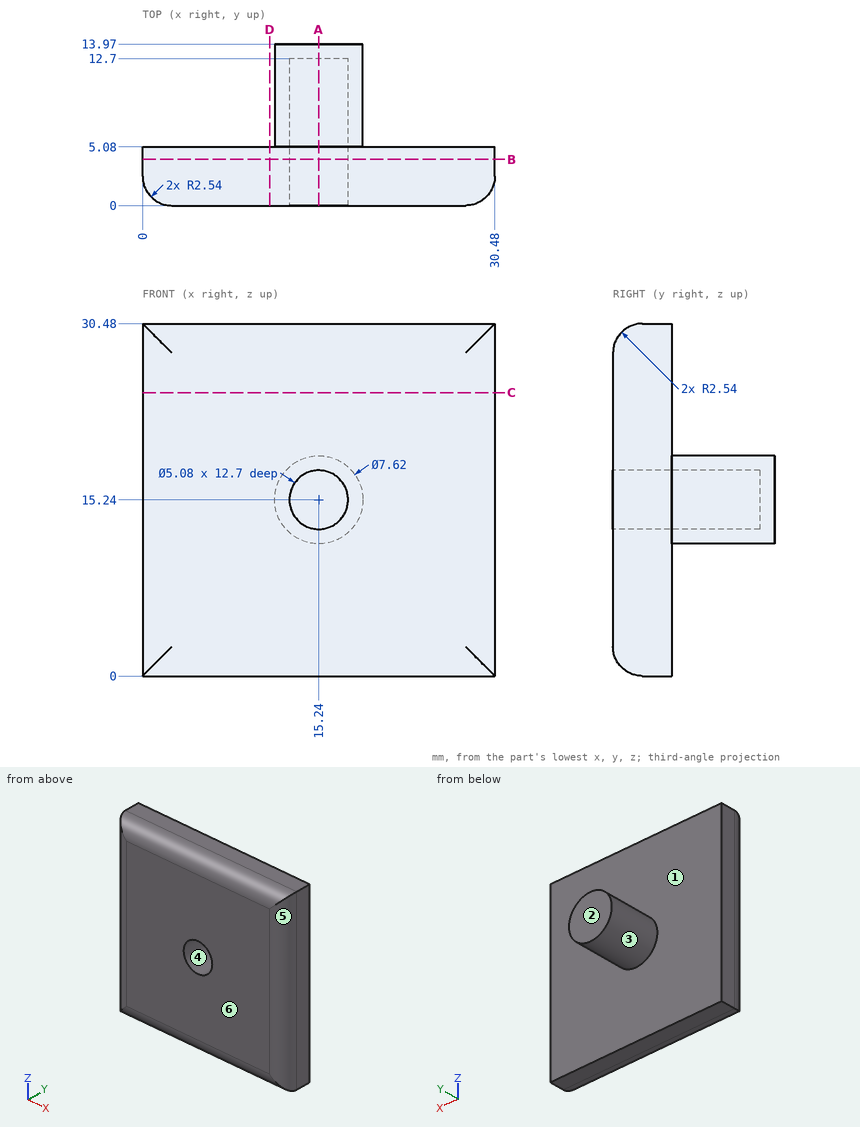
For this review, use the dimensioned drawing (mm, ordinates from the lowest corner) and the shaded views. A direction names the side the tool comes from. Round coordinates to 2 decimals unless told otherwise and drop trailing zeros. Order: outer loops, then holes, each group sorted by start corner. A loop starts at its lowest first (then second) coordinate and runs counter-clockwise, first axis right, second up. Notation, with made-up numbers: M 51.25,1 L 62.25,1 A9 ccw 62.25,13 Z; hole C -40,-24.5 d8. An arc over 180 degrees is marked long. Use a Markdown table: item, result. Add a question column.
Item 1: Insertion check: pin 1 (8 mm diameter, centred on y = 7.5, z = 21.5, fed in from +X); pin 2 (2 mm diameter, centred on y = 11, z = 17.5, fed in from +X); pin 3 (5 mm diameter, centred on x = 3, z = 4, fed in from +Y). Each pin has a flat end and moves straight along its axis. Give the tip position at first contact, or say it passes through.
Item 2: Add section B-B, the plane y = 4. Give the boundary of the cut face in (x, z), then the cut area to 3 significant figures.
Item 3: Add section D-D, the plane x = 11. Give the boundary of the cut face in (y, z).
Item 4: Tool access review of the marked faces 1 and 2: name each direction out of +Z, -Z, +X, -X, +Y, -Y from which nothing blocks a thin tool from reaching the whole face with its end or side.
Item 5: Mouldability with a two-part tool opening along X and no side actions: class the marked faces 3, 4, 5 and 6 as released by +X, released by -X, zero draft, split by the parting line, or undercut.
Item 6: Add section C-C, the plane z = 24.5. Give the boundary of the cut face in (x, y).
Item 7: To check wall thickness, follow line 1 along Z through (x, y) = (15.24, 8.5); line 2 along Y through (x, z) = (6.5, 20.5); line 3 along Z through (x, y) = (13.5, 12.5). State the ranges of each line that lie inside material, in increasing order.
Item 8: Add section A-A, the plane x = 15.24. Give the boundary of the cut face in (y, z), then the cut area to 3 significant figures.
Geometry results:
| question | item | result |
|---|---|---|
| 1 | pin 1 | stops at x = 30.48 |
| 1 | pin 2 | stops at x = 18.84 |
| 1 | pin 3 | stops at y = 5.08 |
| 2 | outline | M 0,0 L 30.48,0 L 30.48,30.48 L 0,30.48 Z; hole C 15.24,15.24 d5.08 |
| 2 | area | 909 mm² |
| 3 | outline | M 0,2.54 A2.54 ccw 2.54,0 L 5.08,0 L 5.08,30.48 L 2.54,30.48 A2.54 ccw 0,27.94 Z |
| 4 | face 1 | +Y |
| 4 | face 2 | +Z, -Z, +X, -X, +Y |
| 5 | face 3 | split by the parting line |
| 5 | face 4 | undercut |
| 5 | face 5 | released by +X |
| 5 | face 6 | zero draft |
| 6 | outline | M 0,2.54 A2.54 ccw 2.54,0 L 27.94,0 A2.54 ccw 30.48,2.54 L 30.48,5.08 L 0,5.08 Z |
| 7 | line 1 | z = 11.43 to 12.7, 17.78 to 19.05 |
| 7 | line 2 | y = 0 to 5.08 |
| 7 | line 3 | z = 11.85 to 13.39, 17.09 to 18.63 |
| 8 | outline | M 0,2.54 A2.54 ccw 2.54,0 L 5.08,0 L 5.08,11.43 L 13.97,11.43 L 13.97,19.05 L 5.08,19.05 L 5.08,30.48 L 2.54,30.48 A2.54 ccw 0,27.94 L 0,17.78 L 12.7,17.78 L 12.7,12.7 L 0,12.7 Z |
| 8 | area | 155 mm² |
